Source: CAD feature listing. Evaluate the final solid. Frame: model axes, mm. A direction names the side the tool comes from. Coordinates: 2 decimals unless noted, no trailing zeros. Write each loop counter-clockwise with the first axis right and the second up, starting at its lowest first coordinate (ties: lowest second). Pieces come first, ordered by that corner, then holes. Notation, with made-up numbers: (28, -9) -> (62, -9) arc R14 ccw to (62, -5) -> close; hole circle Ø4 at (21, -35). An arc over 180 degrees is marked (long way). One line per item, written item: value. Start each with the question number.
1. Access query for faces 4 (the cylindrical face through (-0.86, -1, 105.08)), 5 (the cylindrical face through (-1.8, 3.8, 100.6)). Directions: +Z, -Z, +X, -X, +Y, -Y. A direction counts if a zero-diameter tool reaches every point of the face in a straight line with its end or side. Return the directions, or none.
2. Section query B-B, the plane y = -3.25. Output: boundary loops of the cut face in (x, z), and give its area (3 significant figures).
3. Mould query, pull axis Z, two halves, no side actions, for faces 1 (the flat face through (7.5, -1, 123)), 2 (the cylindrical face through (0.676, -0.998, 17.146)), 3 (the flat face through (0, 0, 0)). Classes: released by +Z, released by -Z, zero draft, split by the parting line, or undercut.
4. Line query: line 1 (Y direction, x = -6.5, z = 131.5); line 2 (X direction, y = -0.25, z = 235); line 3 (Y direction, x = 7, z = 132.5). Output: solid intervals per line, ascending.
5. First-contact query: P1, Ø6.5, axis at x = 0.5, z = 235, coming from the +Y side; P2, Ø5, axis at x = 0, z = 103, coming from the +Y side; P3, Ø0.6, axis at y = 3.5, z = 84.5, coming from the +X side. Flat tips, straight axial feed; report the tip coordinate or a pass-through.
6. Section query C-C, the plane x = 0. State how many separate pieces and enclosed holes the cut face has, and give its area (3 significant figures).
from build123d import *

# Parameters (mm, degrees)
EXTRUDE1_DEPTH             = 250
EXTRUDE2_REACH             = 252.312
SKETCH2_R                  = 2.25
SKETCH_R                   = 3
SKETCH_R_2                 = 2.25
EXTRUDE4_DEPTH             = 2.3
CHAMFER1_SIZE              = 0.2
LPATTERN1_COUNT            = 6
LPATTERN1_PITCH            = 44
CHAMFER1_OF_LPATTERN1_SIZE = 0.2


with BuildPart() as part:
    # Sketch1 → Extrude1 (new body)
    with BuildSketch(Plane.XY):
        with BuildLine():
            Line((-7.3, -5), (7.3, -5))
            Line((7.3, -5), (7.5, -4.8))
            Line((7.5, -4.8), (7.5, 2.706274607))
            ThreePointArc((7.5, 2.706274607), (7.091294745, 2.882570681), (6.840065792, 3.25))
            Line((6.840065792, 3.25), (6.340065792, 3.25))
            Line((6.340065792, 3.25), (6.340065792, 3.75))
            Line((6.340065792, 3.75), (6.840065792, 3.75))
            ThreePointArc((6.840065792, 3.75), (7.091294745, 4.117429319), (7.5, 4.293725393))
            Line((7.5, 4.293725393), (7.5, 4.8))
            Line((7.5, 4.8), (7.3, 5))
            Line((7.3, 5), (-7.3, 5))
            Line((-7.3, 5), (-7.5, 4.8))
            Line((-7.5, 4.8), (-7.5, 4.293725393))
            ThreePointArc((-7.5, 4.293725393), (-7.091294745, 4.117429319), (-6.840065792, 3.75))
            Line((-6.840065792, 3.75), (-6.340065792, 3.75))
            Line((-6.340065792, 3.75), (-6.340065792, 3.25))
            Line((-6.340065792, 3.25), (-6.840065792, 3.25))
            ThreePointArc((-6.840065792, 3.25), (-7.091294745, 2.882570681), (-7.5, 2.706274607))
            Line((-7.5, 2.706274607), (-7.5, -4.8))
            Line((-7.5, -4.8), (-7.3, -5))
        make_face()
    extrude(amount=EXTRUDE1_DEPTH)

    # Sketch2 → Extrude2 (cut, up to next)
    with BuildSketch(Plane(origin=(0, 5, 0), x_dir=(1, 0, 0), z_dir=(0, 1, 0)), mode=Mode.PRIVATE) as extrude2_sk1:
        with Locations(Location((0, -15, 0), (0, 0, 270))):
            Circle(SKETCH2_R)
    extrude2_tool1 = extrude(extrude2_sk1.sketch, amount=-EXTRUDE2_REACH, mode=Mode.PRIVATE) & part.part
    extrude2 = extrude2_tool1.solids().sort_by_distance((0, 5, 15))[0]
    add(extrude2, mode=Mode.SUBTRACT)

    # Sketch → Extrude4 (cut)
    with BuildSketch(Plane(origin=(0, 5, 0), x_dir=(1, 0, 0), z_dir=(0, 1, 0))):
        with Locations(Location((0, -15, 0), (0, 0, 270))):
            Circle(SKETCH_R)
        with Locations(Location((0, -15, 0), (0, 0, 270))):
            Circle(SKETCH_R_2, mode=Mode.SUBTRACT)
    extrude4 = extrude(amount=-EXTRUDE4_DEPTH, mode=Mode.SUBTRACT)

    # Chamfer1
    chamfer1_edges = [part.edges().sort_by_distance(p)[0] for p in [
        (0, -5, 12.75),
        (0, 5, 12),
    ]]
    chamfer(chamfer1_edges, length=CHAMFER1_SIZE)

    # LPattern1: Extrude2, Extrude4 ×6
    with Locations(*[(0, 0, i * LPATTERN1_PITCH) for i in range(1, LPATTERN1_COUNT)]):
        add(extrude2, mode=Mode.SUBTRACT)
        add(extrude4, mode=Mode.SUBTRACT)

    # Chamfer1 of LPattern1
    chamfer1_of_lpattern1_edges = [part.edges().sort_by_distance(p)[0] for p in [
        (0, -5, 56.75),
        (0, 5, 56),
        (0, -5, 100.75),
        (0, 5, 100),
        (0, -5, 144.75),
        (0, 5, 144),
        (0, -5, 188.75),
        (0, 5, 188),
        (0, -5, 232.75),
        (0, 5, 232),
    ]]
    chamfer(chamfer1_of_lpattern1_edges, length=CHAMFER1_OF_LPATTERN1_SIZE)


solid = part.part
Computed values:
1. face 4: +Y, -Y
1. face 5: +Y
2. outline: (-7.5, 0) -> (7.5, 0) -> (7.5, 250) -> (-7.5, 250) -> close; hole circle Ø4.5 at (0, 15); hole circle Ø4.5 at (0, 59); hole circle Ø4.5 at (0, 103); hole circle Ø4.5 at (0, 147); hole circle Ø4.5 at (0, 191); hole circle Ø4.5 at (0, 235)
2. area: 3,650 mm²
3. face 1: zero draft
3. face 2: undercut
3. face 3: released by -Z
4. line 1: y = -5 to 3.25, 3.75 to 5
4. line 2: x = -7.5 to -2.25, 2.25 to 7.5
4. line 3: y = -5 to 2.97, 4.03 to 5
5. P1: stops at y = 5
5. P2: stops at y = 2.7
5. P3: stops at x = 6.86
6. separate pieces: 7
6. enclosed holes: 0
6. area: 2,210 mm²
